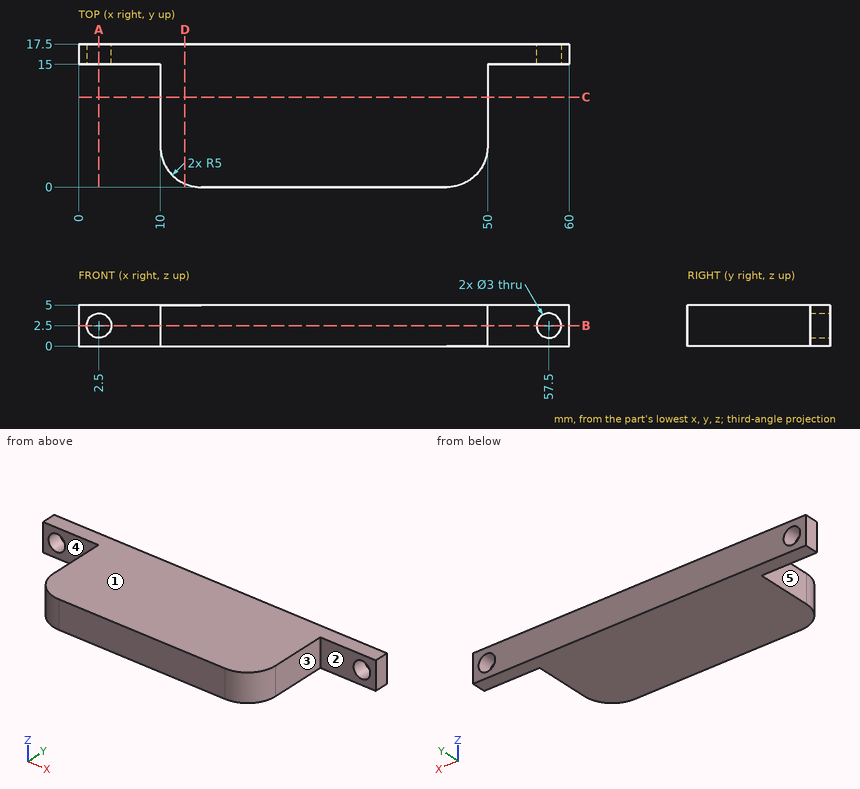
For this review, use the dimensioned drawing (mm, ordinates from the lowest corner) and the shaded views. A direction names the side the tool comes from. Coordinates: 2 decimals unless noted, no trailing zeros. Order: outer loops, then holes, each group sorted by start corner. A loop starts at its lowest first (then second) coordinate and runs counter-clockwise, first axis right, second up. Notation, with made-up numbers: (-11.75, 34) - (-2.75, 34) arc R14 ccw to (-2.75, 60) - close; hole circle Ø2 at (42, 59). An arc over 180 degrees is marked (long way). Answer as a JSON object with one key per item and string values. Group by question number.
1. We need section B-B on z = 2.5. State the section outline as (x, y) points.
2. We need section D-D on x = 13. State the section outline as (y, z) points.
3. We need section A-A on x = 2.5. State the section outline as (y, z) points, then the cut area to 3 significant figures.
4. Clearance check with flat-ended pins moving along their axes: P1, Ø1.5, axis at x = 4.5, z = 2.5, coming from the -Y side; P2, Ø2.5, axis at y = 9.5, z = 2, coming from the -X side; P3, Ø2, axis at y = 3, z = 2.5, coming from the +X side; P4, Ø2.5, axis at x = 2.5, z = 2.5, coming from the +Y side. State where each tip first meets the part, or that it passes through.
5. The part is to be moulded in two halves that separate along X. For the marked faces 3, 4 and 5, say which applies: pulls with the +X half, pulls with the -X half, needs draft (parallel to the pull), parting line crosses it, or undercut.
6. We need section C-C on y = 11. State the section outline as (x, z) points.
7. For the marked faces 1 and 2, list the 3-axis set-ups (+Z, -Z, +X, -X, +Y, -Y) from which the entire face can be reached by the end or side of a thin tool; tool diameter is ignored.
8. For probe 1 along Z at (x, y) = (2.5, 15.55); probe 2 along X at (y, z) = (9, 2.7); probe 3 along Y at (x, z) = (54, 0.65), list the stretches that pass through material, from the lowest coordinate up.
Final values:
{
 "1": {"outline": "(0, 15) - (1, 15) - (1, 17.5) - (0, 17.5) - close; (4, 15) - (10, 15) - (10, 5) arc R5 ccw to (15, 0) - (45, 0) arc R5 ccw to (50, 5) - (50, 15) - (56, 15) - (56, 17.5) - (4, 17.5) - close; (59, 15) - (60, 15) - (60, 17.5) - (59, 17.5) - close"},
 "2": {"outline": "(0.42, 0) - (17.5, 0) - (17.5, 5) - (0.42, 5) - close"},
 "3": {"outline": "(15, 0) - (17.5, 0) - (17.5, 1) - (15, 1) - close; (15, 4) - (17.5, 4) - (17.5, 5) - (15, 5) - close", "area": "5.00 mm²"},
 "4": {"P1": "y = 15", "P2": "x = 10", "P3": "x = 49.9", "P4": "through"},
 "5": {"face 3": "pulls with the +X half", "face 4": "needs draft", "face 5": "pulls with the -X half"},
 "6": {"outline": "(10, 0) - (50, 0) - (50, 5) - (10, 5) - close"},
 "7": {"face 1": "+Z, +X, -X, +Y, -Y", "face 2": "+Z, -Z, +X, -Y"},
 "8": {"probe 1": "0 to 1, 4 to 5", "probe 2": "10 to 50", "probe 3": "15 to 17.5"}
}
